from build123d import *

# Parameters (mm, degrees)
CROQUIS1_W              = 987.3
CROQUIS1_H              = 900
CROQUIS1_W_2            = 911.1
CROQUIS1_H_2            = 823.8
SALIENTE_EXTRUIR1_DEPTH = 3.1
CROQUIS2_W              = 987.3
CROQUIS2_H              = 900
CROQUIS2_W_2            = 981.1
CROQUIS2_H_2            = 893.8
SALIENTE_EXTRUIR2_DEPTH = 38.1
CROQUIS3_R              = 3.175
CORTAR_EXTRUIR1_DEPTH   = 1000


with BuildPart() as part:
    # Croquis1 → Saliente-Extruir1 (new body)
    with BuildSketch(Plane.XY):
        with Locations((-493.65, 450)):
            Rectangle(CROQUIS1_W, CROQUIS1_H)
        with Locations((-493.65, 450)):
            Rectangle(CROQUIS1_W_2, CROQUIS1_H_2, mode=Mode.SUBTRACT)
    extrude(amount=SALIENTE_EXTRUIR1_DEPTH)

    # Croquis2 → Saliente-Extruir2 (add)
    with BuildSketch(Plane.XY.offset(3.1)):
        with Locations((-493.65, 450)):
            Rectangle(CROQUIS2_W, CROQUIS2_H)
        with Locations((-493.65, 450)):
            Rectangle(CROQUIS2_W_2, CROQUIS2_H_2, mode=Mode.SUBTRACT)
    extrude(amount=SALIENTE_EXTRUIR2_DEPTH)

    # Croquis3 → Cortar-Extruir1 (cut)
    with BuildSketch(Plane.ZY.offset(987.3)):
        with Locations((11.075, 859)):
            Circle(CROQUIS3_R)
        with Locations((11.075, 831)):
            Circle(CROQUIS3_R)
        with Locations((30.125, 859)):
            Circle(CROQUIS3_R)
        with Locations((30.125, 831)):
            Circle(CROQUIS3_R)
        with Locations((30.125, 69)):
            Circle(CROQUIS3_R)
        with Locations((11.075, 69)):
            Circle(CROQUIS3_R)
        with Locations((11.075, 41)):
            Circle(CROQUIS3_R)
        with Locations((30.125, 41)):
            Circle(CROQUIS3_R)
    extrude(amount=-CORTAR_EXTRUIR1_DEPTH, mode=Mode.SUBTRACT)


solid = part.part
Model file for the job. Use its own axes, mm. A direction names the side the tool comes from. Coordinates: 2 decimals unless noted, no trailing zeros. Write each loop counter-clockwise with the first axis right and the second up, starting at its lowest first coordinate (ties: lowest second). Pieces come first, ordered by that corner, then holes. Notation, with made-up numbers: (64.5, 70.25) -> (113.5, 70.25) arc R25 ccw to (113.5, 91.25) -> close; hole circle Ø8 at (-19.75, 47.25). An arc over 180 degrees is marked (long way). One line per item, written item: value. Start each with the question number.
1) Which spindle directions (+Z, -Z, +X, -X, +Y, -Y) get a long thin tool onto all of the face, cutting with end or side? Do faces 5 (the face through (-501, 0, 20)), 6 (the face through (-532, 22, 3.1)). Say none if no direction does.
2) Pull direction X, two halves, no side cores. Call faces 1 (the face through (0, 444, 20)), 2 (the face through (-987.3, 444, 20)), 3 (the face through (-501, 900, 20)), 4 (the face through (-3.1, 444, 22)): +X half, -X half, draft (parallel to the pull), parting line (faces both ways), or undercut.
3) Probe probe 1 along Z at (x, y) = (-1.5, 859); probe 2 along Y at (x, z) = (-879, 8.5); probe 3 along Y at (x, z) = (-373, 2.5). List the from-to ranges inside material, lowest first.
4) Slice it at A-A on y = 256. Write the cut outline in (x, z), then the cut area to 3 significant figures.
5) Flat gauge pin, fed straight in: pin 1 Ø5.5 at (y, z) = (69, 11.075) entering from -X. Where does the tip first touch, or does it go through?
6) Slice it at B-B on x = -653. Write the cut outline in (y, z).
Answers follow:
1. face 5: +Z, -Z, +X, -X, -Y
1. face 6: +Z
2. face 1: +X half
2. face 2: -X half
2. face 3: draft
2. face 4: undercut
3. probe 1: 0 to 7.9, 14.25 to 26.95, 33.3 to 41.2
3. probe 2: 0 to 3.1, 896.9 to 900
3. probe 3: 0 to 38.1, 861.9 to 900
4. outline: (-987.3, 0) -> (-949.2, 0) -> (-949.2, 3.1) -> (-984.2, 3.1) -> (-984.2, 41.2) -> (-987.3, 41.2) -> close; (-38.1, 0) -> (0, 0) -> (0, 41.2) -> (-3.1, 41.2) -> (-3.1, 3.1) -> (-38.1, 3.1) -> close
4. area: 472 mm2
5. pin 1: through
6. outline: (0, 0) -> (38.1, 0) -> (38.1, 3.1) -> (3.1, 3.1) -> (3.1, 41.2) -> (0, 41.2) -> close; (861.9, 0) -> (900, 0) -> (900, 41.2) -> (896.9, 41.2) -> (896.9, 3.1) -> (861.9, 3.1) -> close
